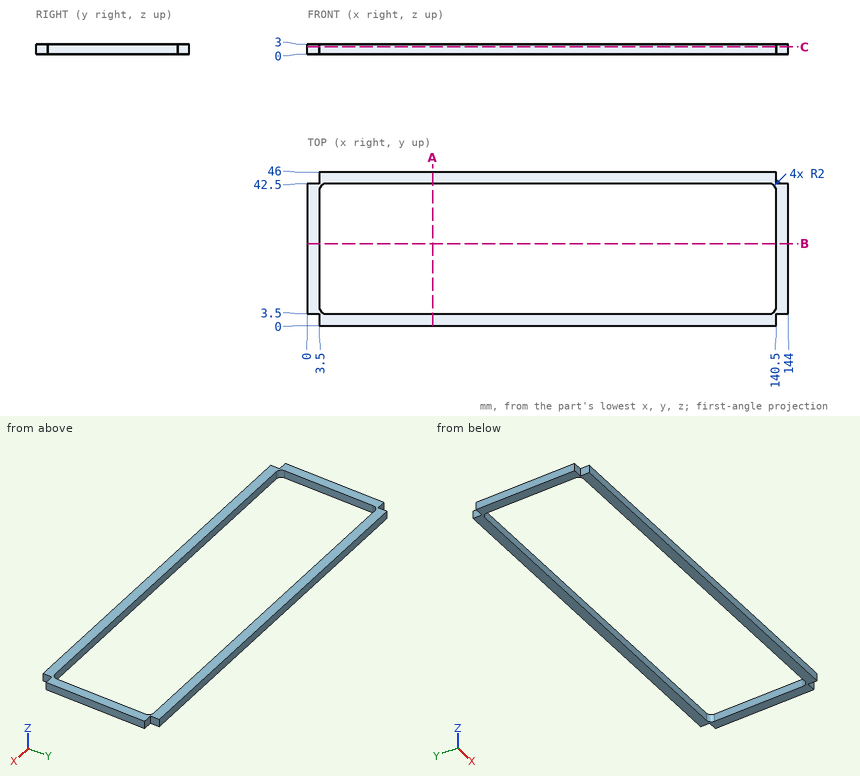
For this review, use the dimensioned drawing (mm, ordinates from the lowest corner) and the shaded views. Coordinates: 2 decimals unless noted, no trailing zeros. Order: outer loops, then holes, each group sorted by start corner. A loop starts at its lowest first (then second) coordinate and runs counter-clockwise, first axis right, second up. Notation, with made-up numbers: (56.5, 6) - (62.5, 6) arc R29 ccw to (62.5, 26) - close; hole circle Ø5 at (57, -6). An arc over 180 degrees is marked (long way). Answer in a Markdown table with one row per item.
(1) Consider section B-B on y = 24.5. State the section outline as (x, z) points, plus the area to 3 significant figures.
Checked values:
| item | result |
|---|---|
| outline | (0, 0) - (3.5, 0) - (3.5, 3) - (0, 3) - close; (140.5, 0) - (144, 0) - (144, 3) - (140.5, 3) - close |
| area | 21.0 mm^2 |
(2) Wall thickness on line 1 along X through (y, z) = (37, 0.4); line 2 along Y through (x, z) = (39, 1.55); line 3 along X through (y, z) = (43.5, 2.5): over which ranges is each line inside the solid? List them lowest first. Write a range as from..to.
Checked values:
| item | result |
|---|---|
| line 1 | 0..3.5, 140.5..144 |
| line 2 | 0..3.5, 42.5..46 |
| line 3 | 3.5..140.5 |
(3) Clearance check with flat-ended pins moving along their axes: pin 1 (0.9 mm diameter, centred on x = 142, z = 1.5, fed in from +Y); pin 2 (1.5 mm diameter, centred on y = 2, z = 1, fed in from +X); pin 3 (1.5 mm diameter, centred on x = 142, z = 1, fed in from -Y); pin 4 (3 mm diameter, centred on x = 54.5, y = 40, fed in from -Z). State where each tip first meets the part, or that it passes through.
Checked values:
| item | result |
|---|---|
| pin 1 | y = 42.5 |
| pin 2 | x = 140.5 |
| pin 3 | y = 3.5 |
| pin 4 | through |
(4) Consider section C-C on z = 2.15. State the section outline as (x, y) points.
Checked values:
| item | result |
|---|---|
| outline | (0, 3.5) - (3.5, 3.5) - (3.5, 0) - (140.5, 0) - (140.5, 3.5) - (144, 3.5) - (144, 42.5) - (140.5, 42.5) - (140.5, 46) - (3.5, 46) - (3.5, 42.5) - (0, 42.5) - close; hole (3.5, 5.5) arc R2 ccw to (5.5, 3.5) - (138.5, 3.5) arc R2 ccw to (140.5, 5.5) - (140.5, 40.5) arc R2 ccw to (138.5, 42.5) - (5.5, 42.5) arc R2 ccw to (3.5, 40.5) - close |
(5) Consider section A-A on x = 37.5. State the section outline as (y, z) points, plus the area to 3 significant figures.
Checked values:
| item | result |
|---|---|
| outline | (0, 0) - (3.5, 0) - (3.5, 3) - (0, 3) - close; (42.5, 0) - (46, 0) - (46, 3) - (42.5, 3) - close |
| area | 21.0 mm^2 |
